Design review of the part built by this model. Coordinates are the model's own, in mm. Round coordinates to 2 decimals unless told otherwise and drop trailing zeros. Order: outer loops, then holes, each group sorted by start corner. A loop starts at its lowest first (then second) coordinate and runs counter-clockwise, first axis right, second up.
from build123d import *

# Parameters (mm, degrees)
F0_R     = 6.35
F1_DEPTH = 31.75
F2_R     = 6.35
F3_DEPTH = 44.45
F5_DEPTH = 31.75


with BuildPart() as f1:
    # F0 (on Top) → F1 (new body)
    with BuildSketch(Plane.XY):
        with BuildLine():
            Line((1016, 120.65), (0, 120.65))
            ThreePointArc((0, 120.65), (-120.65, 0), (0, -120.65))
            Line((0, -120.65), (1016, -120.65))
            Line((1016, -120.65), (1016, 120.65))
        make_face()
        Circle(F0_R, mode=Mode.SUBTRACT)
    extrude(amount=F1_DEPTH)

    # F2 (on face) → F3 (join)
    with BuildSketch(Plane(origin=(0, 0, 0), x_dir=(1, 0, 0), z_dir=(0, 0, -1))):
        with Locations((279.4, 114.3)):
            Circle(F2_R)
    extrude(amount=F3_DEPTH)

    # F4 (on face) → F5 (cut)
    with BuildSketch(Plane(origin=(0, 0, 0), x_dir=(1, 0, 0), z_dir=(0, 0, -1))):
        with BuildLine():
            Line((286.004, -120.65), (286.004, -114.046))
            ThreePointArc((286.004, -114.046), (279.4, -107.442), (272.796, -114.046))
            Line((272.796, -114.046), (272.796, -120.65))
            Line((272.796, -120.65), (286.004, -120.65))
        make_face()
    extrude(amount=-F5_DEPTH, mode=Mode.SUBTRACT)


solid = f1.part
1) Take a section at C-C on y = -63. Give the boundary of the cut face in (x, z), plus the area to 3 significant figures.
Results:
outline: (-102.9, 0) - (1016, 0) - (1016, 31.75) - (-102.9, 31.75) - close
area: 35,500 mm2
2) Take a section at A-A on z = 14. Give the boundary of the cut face in (x, y), plus the area to 3 significant figures.
Results:
outline: (0, -120.65) - (1016, -120.65) - (1016, 120.65) - (286, 120.65) - (286, 114.05) arc R6.6 cw to (272.8, 114.05) - (272.8, 120.65) - (0, 120.65) arc R120.65 ccw to start; hole circle Ø12.7 at (0, 0)
area: 268,000 mm2
3) To check wall thickness, follow line 1 along Y through (x, z) = (0, 10); line 2 along Z through (x, y) = (108, 3); line 3 along Y through (x, z) = (-3, 17.5). State the ranges of each line that lie inside material, in increasing order.
Results:
line 1: y = -120.65 to -6.35, 6.35 to 120.65
line 2: z = 0 to 31.75
line 3: y = -120.61 to -5.6, 5.6 to 120.61
4) Clearance check with flat-ended pins moving along their axes: P1, Ø8, axis at x = 406.5, y = -76.5, coming from the -Z side; P2, Ø7.5, axis at x = 0, y = 0, coming from the -Z side; P3, Ø12, axis at y = -60.5, z = 10.5, coming from the -X side. State where each tip first meets the part, or that it passes through.
Results:
P1: stops at z = 0
P2: passes through
P3: stops at x = -107.64
5) Take a section at B-B on x = 127. Give the boundary of the cut face in (y, z), plus the area to 3 significant figures.
Results:
outline: (-120.65, 0) - (120.65, 0) - (120.65, 31.75) - (-120.65, 31.75) - close
area: 7,660 mm2
